```python
from build123d import *

# Parameters (mm, degrees)
SKETCH1_W           = 96
SKETCH1_H           = 40
SKETCH1_R           = 1.5
SKETCH1_W_2         = 25
SKETCH1_H_2         = 25
SKETCH1_W_3         = 41
BOSS_EXTRUDE1_DEPTH = 5
FILLET1_R           = 5


with BuildPart() as part:
    # Sketch1 → Boss-Extrude1 (new body)
    with BuildSketch(Plane(origin=(0, 0, 0), x_dir=(1, 0, 0), z_dir=(0, 1, 0))):
        with Locations((8, 0)):
            Rectangle(SKETCH1_W, SKETCH1_H)
        with Locations((-35, 15)):
            Circle(SKETCH1_R, mode=Mode.SUBTRACT)
        with Locations((0, 15)):
            Circle(SKETCH1_R, mode=Mode.SUBTRACT)
        with Locations((50.997548961, -15.5)):
            Circle(SKETCH1_R, mode=Mode.SUBTRACT)
        with Locations((50.997548961, 15.5)):
            Circle(SKETCH1_R, mode=Mode.SUBTRACT)
        with Locations((-35, -15)):
            Circle(SKETCH1_R, mode=Mode.SUBTRACT)
        with Locations((0, -15)):
            Circle(SKETCH1_R, mode=Mode.SUBTRACT)
        with Locations((-18, 0)):
            Rectangle(SKETCH1_W_2, SKETCH1_H_2, mode=Mode.SUBTRACT)
        with Locations((26, 0)):
            Rectangle(SKETCH1_W_3, SKETCH1_H_2, mode=Mode.SUBTRACT)
    extrude(amount=BOSS_EXTRUDE1_DEPTH)

    # Fillet1
    fillet1_edges = [part.edges().sort_by_distance(p)[0] for p in [
        (-5.5, 2.5, 12.5),
        (-5.5, 2.5, -12.5),
        (-30.5, 2.5, -12.5),
        (-30.5, 2.5, 12.5),
        (-40, 2.5, 20),
        (-40, 2.5, -20),
        (56, 2.5, -20),
        (56, 2.5, 20),
        (46.5, 2.5, 12.5),
        (46.5, 2.5, -12.5),
        (5.5, 2.5, -12.5),
        (5.5, 2.5, 12.5),
    ]]
    fillet(fillet1_edges, radius=FILLET1_R)


solid = part.part
```
The listing builds one solid part. Answer for the finished solid, in the listing's coordinates (mm). A direction names the side the tool comes from. Give positions to 0.01 mm unless a question says otherwise; leave off trailing zeros. Order: outer loops, then holes, each group sorted by start corner. A loop starts at its lowest first (then second) coordinate and runs counter-clockwise, first axis right, second up. Notation, with made-up numbers: (36.25, -26.5) -> (59.25, -26.5) arc R17 ccw to (59.25, -11.5) -> close; hole circle Ø2 at (-13.5, 8.5). An arc over 180 degrees is marked (long way). Write each question's results on one line, items separated by ' | '.
Q1. The part is cut by section D-D, the plane y = 2.5. State how many separate pieces and enclosed holes the cut face has, and give its area (3 significant figures).
Checked values:
separate pieces: 1 | enclosed holes: 8 | area: 2,170 mm^2
Q2. Determine the mould class of faces 1 (the face through (-6.93, 2.54, -11)), 2 (the face through (7, 2, 20)), 3 (the face through (7, 2, -20)) for opening direction Z: pulls with the +Z half, pulls with the -Z half, needs draft (parallel to the pull), parting line crosses it, or undercut.
Checked values:
face 1: undercut | face 2: pulls with the +Z half | face 3: pulls with the -Z half
Q3. The part is cut by section B-B, the plane x = 0. Give the vertices of the cut face in (y, z).
Checked values:
outline: (0, -20) -> (5, -20) -> (5, -16.5) -> (0, -16.5) -> close; (0, -13.5) -> (5, -13.5) -> (5, 13.5) -> (0, 13.5) -> close; (0, 16.5) -> (5, 16.5) -> (5, 20) -> (0, 20) -> close
Q4. This flat-tipped pin is pushed along its axis until it touches: P1, Ø2.5, axis at x = 0, z = 15, coming from the -Y side. Where does it stop, or does it pass through?
Checked values:
P1: passes through
Q5. Straight lines are drawn through the part: probe 1 along Z at (x, y) = (0, 2.4); probe 2 along X at (y, z) = (0.85, -7.5); probe 3 along X at (y, z) = (1.3, -15.5). For each, find the intervals that lie inside material, in ascending order. Write a range as from..to.
Checked values:
probe 1: z = -20..-16.5, -13.5..13.5, 16.5..20 | probe 2: x = -40..-30.5, -5.5..5.5, 46.5..56 | probe 3: x = -39.97..-36.41, -33.59..-1.41, 1.41..49.5, 52.5..55.97
Q6. Which of the six approach directions +Z, -Z, +X, -X, +Y, -Y give full straight-line access (tool end or side, diameter ignored) to faces 4 (the face through (54, 3, 19)), 5 (the face through (45.07, 2.54, -11))?
Checked values:
face 4: +Z, +X, +Y, -Y | face 5: +Y, -Y
Q7. The part is cut by section C-C, the plane z = 5. Give the vertices of the cut face in (x, y), and give its area (3 significant figures).
Checked values:
outline: (-40, 0) -> (-30.5, 0) -> (-30.5, 5) -> (-40, 5) -> close; (-5.5, 0) -> (5.5, 0) -> (5.5, 5) -> (-5.5, 5) -> close; (46.5, 0) -> (56, 0) -> (56, 5) -> (46.5, 5) -> close | area: 150 mm^2
Q8. The part is cut by section A-A, the plane x = -12. Give the vertices of the cut face in (y, z), and give its area (3 significant figures).
Checked values:
outline: (0, -20) -> (5, -20) -> (5, -12.5) -> (0, -12.5) -> close; (0, 12.5) -> (5, 12.5) -> (5, 20) -> (0, 20) -> close | area: 75.0 mm^2
